The model under review builds one solid part; all positions refer to its coordinate system, in mm. A direction names the side the tool comes from. Coordinates: 2 decimals unless noted, no trailing zeros. Order: outer loops, then holes, each group sorted by start corner. A loop starts at its lowest first (then second) coordinate and runs counter-clockwise, first axis right, second up.
```python
from build123d import *

# Parameters (mm, degrees)
F1_DEPTH = 25.4
F3_DEPTH = 25.4


with BuildPart() as f1:
    # F0 (on Front) → F1 (new body)
    with BuildSketch(Plane.XZ):
        with BuildLine():
            Line((0, 52.337721), (-113.883786, 51.742114))
            Line((-113.883786, 51.742114), (-113.883786, -152.551606))
            Line((-113.883786, -152.551606), (0, -152.551606))
            ThreePointArc((0, -152.551606), (63.101704, -109.526382), (30.253483, -40.577203))
            ThreePointArc((30.253483, -40.577203), (50.728837, 17.472448), (0, 52.337721))
        make_face()
    extrude(amount=F1_DEPTH)

    # F2 (on face) → F3 (cut)
    with BuildSketch(Plane.XZ.offset(25.4)):
        with BuildLine():
            ThreePointArc((-65.174758, -13.412004), (-8.402959, 2.085997), (-65.174758, 17.583998))
            Line((-65.174758, 17.583998), (-65.174758, -13.412004))
        make_face()
        with BuildLine():
            ThreePointArc((-65.174758, -125.446111), (-11.516542, -100.415442), (-65.174758, -75.384773))
            Line((-65.174758, -75.384773), (-65.174758, -125.446111))
        make_face()
    extrude(amount=-F3_DEPTH, mode=Mode.SUBTRACT)


solid = f1.part
```
(1) Draft analysis for pull direction X (two halves, no side actions). For faces 1 (the face through (-65.175, -13, 2)), 2 (the face through (-58, -13, -152.552)), 3 (the face through (-113.884, -13, -49)), 4 (the face through (-8.423, -12.878, 0.972)), state which applies: released by +X, released by -X, zero draft, split by the parting line, or undercut.
A:
face 1: undercut
face 2: zero draft
face 3: released by -X
face 4: undercut
(2) For pin 1 Ø5 at (x, y) = (-18, -10) entering from +Z; pin 2 Ø12.5 at (y, z) = (-18.5, -4.5) entering from +X; pin 3 Ø3 at (y, z) = (-17.5, -51.5) entering from +X, all flat-tipped, find the tip position at first contact; note any pin that passes through.
A:
pin 1: stops at z = 52.26
pin 2: stops at x = 53.21
pin 3: stops at x = 48.22
(3) We need section C-C, the plane x = 45. Write out the cut boundary in (y, z), and give its area (3 significant figures).
A:
outline: (-25.4, -138.47) - (0, -138.47) - (0, -49.97) - (-25.4, -49.97) - close; (-25.4, -25.83) - (0, -25.83) - (0, 29.44) - (-25.4, 29.44) - close
area: 3,650 mm2
(4) Wall thickness on probe 1 along Z at (x, y) = (-14, -9.25); probe 2 along Z at (x, y) = (-53.5, -18.25); probe 3 along X at (y, z) = (-18.5, -72): over which ranges is each line inside the solid? List them lowest first.
A:
probe 1: z = -152.55 to -112.91, -87.92 to -15.52, 19.7 to 52.26
probe 2: z = -152.55 to -131.73, -69.1 to -24.7, 28.87 to 52.06
probe 3: x = -113.88 to -60.3, -28.07 to 60.76
(5) We need section B-B, the plane z = 3. Write out the cut boundary in (x, y), and give its area (3 significant figures).
A:
outline: (-113.88, -25.4) - (-65.17, -25.4) - (-65.17, 0) - (-113.88, 0) - close; (-8.42, -25.4) - (53.2, -25.4) - (53.2, 0) - (-8.42, 0) - close
area: 2,800 mm2
(6) Machinability: for faces 5 (the face through (-65.175, -13, -100)), 6 (the face through (-26, 0, -49)), which of the approach directions +Z, -Z, +X, -X, +Y, -Y give a long, thin tool a straight path to every point of the face, cutting with its end or side? Answer none if there is none.
A:
face 5: +Y, -Y
face 6: +Z, -Z, +X, -X, +Y
(7) We need section A-A, the plane x = -31.5. Write out the cut boundary in (y, z).
A:
outline: (-25.4, -152.55) - (0, -152.55) - (0, -130.52) - (-25.4, -130.52) - close; (-25.4, -70.31) - (0, -70.31) - (0, -27.5) - (-25.4, -27.5) - close; (-25.4, 31.67) - (0, 31.67) - (0, 52.17) - (-25.4, 52.17) - close
(8) We need section D-D, the plane y = -3.25. Write out the cut boundary in (x, z).
A:
outline: (-113.88, -152.55) - (0, -152.55) arc R58.69 ccw to (30.25, -40.58) arc R50.6 ccw to (0, 52.34) - (-113.88, 51.74) - close; hole (-65.17, -125.45) arc R32.67 ccw (long way) to (-65.17, -75.38) - close; hole (-65.17, -13.41) arc R30.5 ccw (long way) to (-65.17, 17.58) - close
